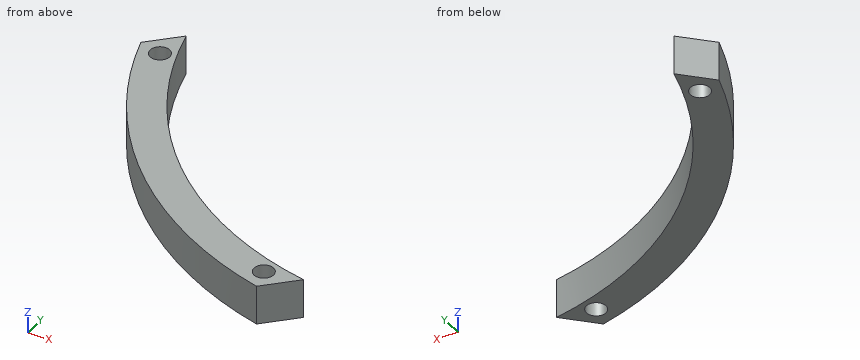
Autodesk Inventor part; units mm, degrees
ref_plane "YZ Plane" through (0, 0, 0) normal (1, 0, 0) x (0, 1, 0)
ref_plane "XZ Plane" through (0, 0, 0) normal (0, 1, 0) x (-1, 0, 0)
ref_plane "XY Plane" through (0, 0, 0) normal (0, 0, 1) x (1, 0, 0)
sketch "Sketch1" plane through (0, 0, 0) normal (0, 0, 1) x (1, 0, 0)
  line L0 (-86.8355, 0) -> (77.4434, 0)
  line L1 (0, -88.2763) -> (0, 77.6836)
  circle A0 centre (0, 0) radius 53.975 construction
  line L2 (-53.2759, -12.7) -> (-57.8106, -17.2347)
  line L3 (-9.2461, -53.9826) -> (-13.9527, -58.6892)
  arc A1 (-53.2759, -12.7) -> (-9.2461, -53.9826) centre (0, 0) ccw
  arc A2 (-57.8106, -17.2347) -> (-13.9527, -58.6892) centre (0, 0) ccw
  point P0 (-54.2025, -18.1167)
  point P1 (-14.9213, -55.1677)
  dimension "d16" = 107.95
  dimension "d17" = 60.325
  dimension "d18" = 5.5563
  dimension "d19" = 0.7937
  dimension "d20" = 3.175
  dimension "d21" = 3.175
  dimension "d22" = 57.15
  dimension "d23" = 57.15
  dimension "d24" = 45
  dimension "d25" = 12.7
extrude "Extrusion1" add sketch "Sketch1" along normal blind 6.35
sketch "Sketch2" plane through (0, 0, 6.35) normal (0, 0, 1) x (1, 0, 0)
  circle A0 centre (0, 0) radius 53.975 construction
  arc A1 (-57.8106, -17.2347) -> (-13.9527, -58.6892) centre (0, 0) ccw
  line L0 (-57.8106, -17.2347) -> (-53.2759, -12.7)
  arc A2 (-53.2759, -12.7) -> (-9.2461, -53.9826) centre (0, 0) ccw
  line L1 (-9.2461, -53.9826) -> (-13.9527, -58.6892)
  line L2 (0, -88.9565) -> (0, 77.7969)
  line L3 (-87.5032, 0) -> (77.5547, 0)
  point P0 (-14.9213, -55.1677)
  point P1 (-54.2025, -18.1167)
  dimension "d27" = 107.95
  dimension "d33" = 57.15
  dimension "d34" = 57.15
  dimension "d37" = 3.175
  dimension "d38" = 3.175
hole "Hole1" at (-54.2025, -18.1167, 6.35) at (-14.9213, -55.1677, 6.35) direction (0, 0, -1) diameter 3.175 end through all
properties part number "motor stay bottom"
CAD build for the part. Positions are in the model's coordinates, mm. Coordinates: 2 decimals unless noted, no trailing zeros. Write each loop counter-clockwise with the first axis right and the second up, starting at its lowest first coordinate (ties: lowest second). Pieces come first, ordered by that corner, then holes. Notation, with made-up numbers: (65, 80.25) - (101, 80.25) arc R21 cw to (101, 111.25) - close; hole circle Ø8 at (9, -7.5). An arc over 180 degrees is marked (long way). Use a Markdown table: item, result. Add a question column.
Item 1: Band-saw the part on B-B, the plane x = -25. Give the cut face in (y, z).
Item 2: Drill centre lines: L1, parallel to Y at x = -14.5, z = 5.5; L2, parallel to Y at x = -16, z = 2.75; L3, parallel to Y at x = -48, z = 4.25. Where is each one in solid material? Low to high. Write a range as from..to.
Item 3: Flat gauge pins, fed straight in: pin 1 (1 mm diameter, centred on x = -44.5, z = 5.5, fed in from +Y); pin 2 (1.5 mm diameter, centred on x = -30, z = 2, fed in from -Y); pin 3 (1 mm diameter, centred on x = -17, z = 2, fed in from +Y). Where does each tip first touch, or does it go through?
Item 4: Band-saw the part on C-C, the plane y = -39. Give the cut face in (x, z).
Item 5: Band-saw the part on A-A, the plane z = 1.5. Give the cut face in (x, y) (1 decimal).
Numbers:
| question | item | result |
|---|---|---|
| 1 | outline | (-54.9, 0) - (-48.73, 0) - (-48.73, 6.35) - (-54.9, 6.35) - close |
| 2 | L1 | -58.56..-56.7, -53.64..-52.81 |
| 2 | L2 | -58.16..-56.33, -54..-52.38 |
| 2 | L3 | -36.54..-26.37 |
| 3 | pin 1 | y = -31.22 |
| 3 | pin 2 | y = -52.76 |
| 3 | pin 3 | y = -51.9 |
| 4 | outline | (-46.02, 0) - (-38.45, 0) - (-38.45, 6.35) - (-46.02, 6.35) - close |
| 5 | outline | (-57.8, -17.2) arc R60.3 ccw to (-14, -58.7) - (-9.2, -54) arc R54.8 cw to (-53.3, -12.7) - close; hole circle Ø3.2 at (-54.2, -18.1); hole circle Ø3.2 at (-14.9, -55.2) |
